```python
from build123d import *

# Parameters (mm, degrees)
SKETCH1_R           = 4.95
BOSS_EXTRUDE1_DEPTH = 37.5
SKETCH2_R           = 7.45
BOSS_EXTRUDE2_DEPTH = 2.5
SKETCH3_R           = 7.45
BOSS_EXTRUDE3_DEPTH = 2.5


with BuildPart() as part:
    # Sketch1 → Boss-Extrude1 (new body)
    with BuildSketch(Plane.XY):
        Circle(SKETCH1_R)
    extrude(amount=BOSS_EXTRUDE1_DEPTH)

    # Sketch2 → Boss-Extrude2 (add)
    with BuildSketch(Plane(origin=(0, 0, 0), x_dir=(-1, 0, 0), z_dir=(0, 0, -1))):
        Circle(SKETCH2_R)
    extrude(amount=BOSS_EXTRUDE2_DEPTH)

    # Sketch3 → Boss-Extrude3 (add)
    with BuildSketch(Plane.XY.offset(37.5)):
        Circle(SKETCH3_R)
    extrude(amount=BOSS_EXTRUDE3_DEPTH)


solid = part.part
```
Can you work these out from the model? Positions are in its coordinate system, mm. A direction names the side the tool comes from. Give positions to 0.01 mm unless a question says otherwise; leave off trailing zeros. Order: outer loops, then holes, each group sorted by start corner. A loop starts at its lowest first (then second) coordinate and runs counter-clockwise, first axis right, second up. Notation, with made-up numbers: (-12, 63) - (18, 63) arc R13 cw to (18, 72) - close; hole circle Ø7 at (-30.75, 33.5). An arc over 180 degrees is marked (long way). Use a Markdown table: item, result. Add a question column.
Q1. Please list where these lines run through material, in increasing order: line 1 along Z through (x, y) = (-1.25, -5); line 2 along Y through (x, z) = (0, 18); line 3 along Y through (x, z) = (4.5, 4.5).
Q2. If we section it at A-A on x = 0: Write out the boundary of the cut face in (y, z).
Q3. I'm going to push flat-ended pins straight in: pin 1 (3 mm diameter, centred on y = -3.5, z = 18.5, fed in from -X); pin 2 (4 mm diameter, centred on y = 3, z = 25, fed in from +X). Where does each tip first touch, or does it pass through?
Q4. On a 3-axis mill with a long thin cutter (end or side, diameter ignored), from which of +Z, -Z, +X, -X, +Y, -Y can I reach the whole of each face in a straight line? I mean faces 5 (the flat face through (-2, -5, 0)), 6 (the cylindrical face through (7.106, 2.238, 38.732)). Say none if no direction works.
Q5. If we section it at C-C on z = 26: Write out the boundary of the cut face in (x, y), plus the area to 3 significant figures.
Q6. If we mould it in two halves opening along Z, with no side actions, what happens to faces 1 (the cylindrical face through (4.72, 1.49, 18.49)), 2 (the flat face through (0, 0, 40)), 3 (the flat face through (0, 0, -2.5)), 4 (the cylindrical face through (-7.106, 2.238, -1.232))? For each: released by +Z, released by -Z, zero draft, split by the parting line, or undercut.
Answers follow:
| question | item | result |
|---|---|---|
| 1 | line 1 | z = -2.5 to 0, 37.5 to 40 |
| 1 | line 2 | y = -4.95 to 4.95 |
| 1 | line 3 | y = -2.06 to 2.06 |
| 2 | outline | (-7.45, -2.5) - (7.45, -2.5) - (7.45, 0) - (4.95, 0) - (4.95, 37.5) - (7.45, 37.5) - (7.45, 40) - (-7.45, 40) - (-7.45, 37.5) - (-4.95, 37.5) - (-4.95, 0) - (-7.45, 0) - close |
| 3 | pin 1 | stops at x = -4.53 |
| 3 | pin 2 | stops at x = 4.85 |
| 4 | face 5 | none |
| 4 | face 6 | +Z, -Z |
| 5 | outline | circle Ø9.9 at (0, 0) |
| 5 | area | 77.0 mm^2 |
| 6 | face 1 | undercut |
| 6 | face 2 | released by +Z |
| 6 | face 3 | released by -Z |
| 6 | face 4 | zero draft |
